Input: dimensioned drawing with shaded views. Units: mm. Origin: part minimum x, y, z. Give positions to 0.01 mm unless a question says otherwise; leave off trailing zeros. Write each loop counter-clockwise with the first axis right and the second up, starting at its lowest first coordinate (ties: lowest second). Pieces come first, ordered by that corner, then holes. Notation, with made-up numbers: M 71,57 L 77,57 A25 cw 77,89 Z; hole C 44,33 d1. An arc over 180 degrees is marked long. Answer as a JSON object with one key per item and string values.
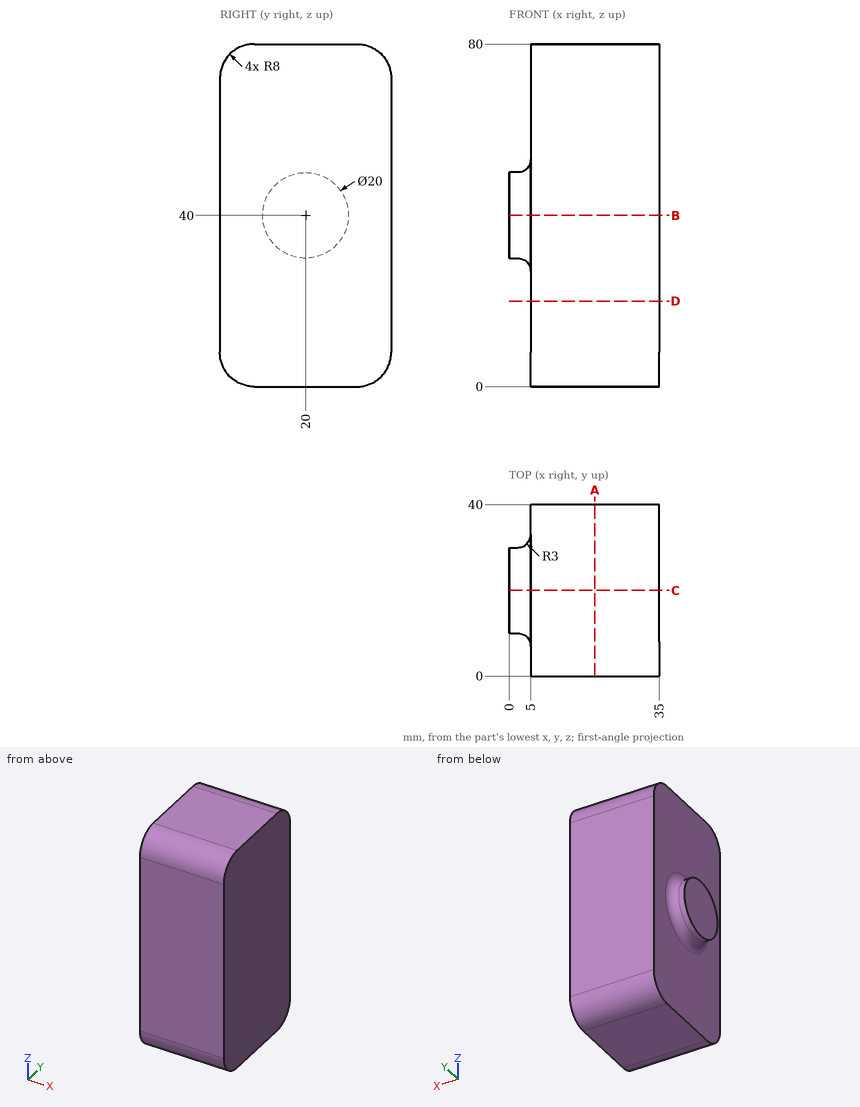
1) Line query: line 1 (X direction, y = 26, z = 55); line 2 (Z direction, x = 9, y = 5.5); line 3 (Y direction, x = 25, z = 7). Output: solid intervals per line, ascending. Write a range as from..to.
Geometry check:
{"line 1": "x = 5..35", "line 2": "z = 0.4..79.6", "line 3": "y = 0.06..39.94"}
2) Cut plane A-A on x = 20. Return loops of the section in (y, z).
Geometry check:
{"outline": "M 0,8 A8 ccw 8,0 L 32,0 A8 ccw 40,8 L 40,72 A8 ccw 32,80 L 8,80 A8 ccw 0,72 Z"}
3) Cut plane D-D on z = 20. Return loops of the section in (x, y).
Geometry check:
{"outline": "M 5,0 L 35,0 L 35,40 L 5,40 Z"}
4) Contact query for flat-ended pins moving along their axis: P1, Ø1, axis at x = 7, y = 25, coming from the -Z side; P2, Ø12, axis at y = 10.5, z = 26, coming from the -X side; P3, Ø2, axis at y = 13, z = 21, coming from the -X side. Output: stop coordinate, or through.
Geometry check:
{"P1": "stops at z = 0", "P2": "stops at x = 4.16", "P3": "stops at x = 5"}
5) Cut plane C-C on y = 20. Return loops of the section in (x, z).
Geometry check:
{"outline": "M 0,30 L 2,30 A3 cw 5,27 L 5,0 L 35,0 L 35,80 L 5,80 L 5,53 A3 cw 2,50 L 0,50 Z"}
6) Cut plane B-B on z = 40. Return loops of the section in (x, y), and give its area (3 significant figures).
Geometry check:
{"outline": "M 0,10 L 2,10 A3 cw 5,7 L 5,0 L 35,0 L 35,40 L 5,40 L 5,33 A3 cw 2,30 L 0,30 Z", "area": "1,300 mm2"}
